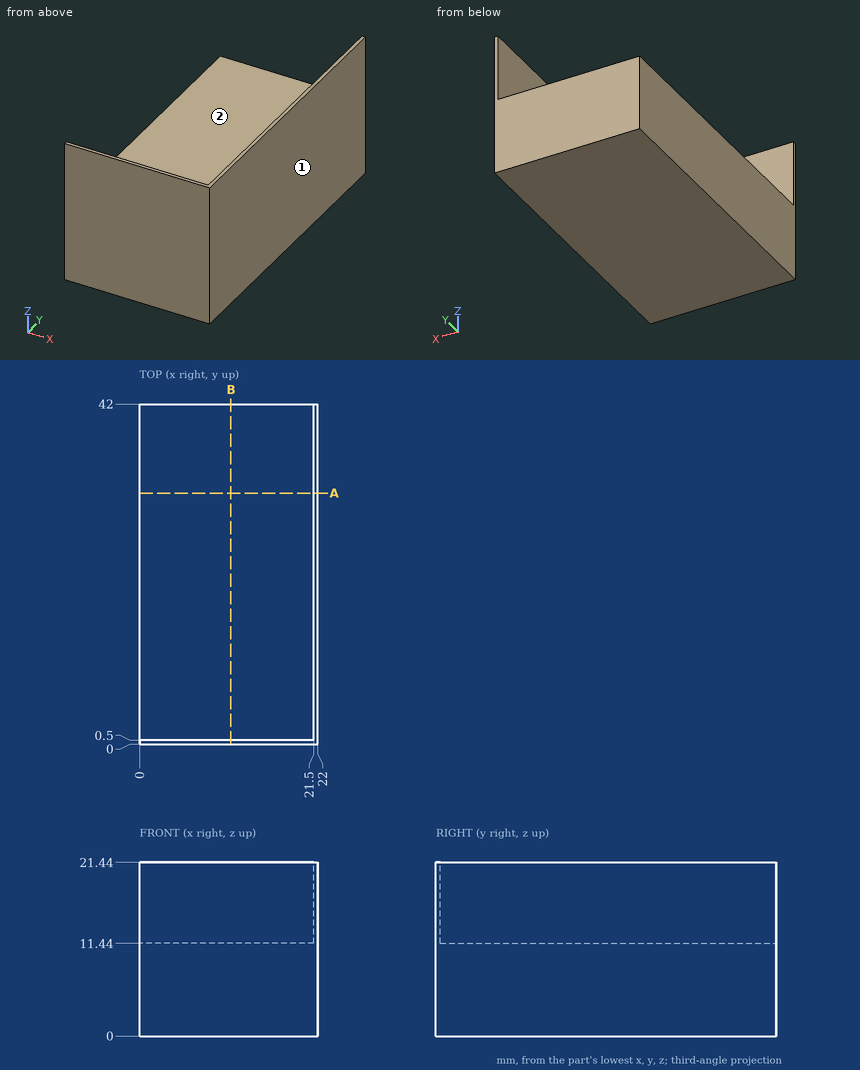
Input: dimensioned drawing with shaded views. Units: mm. Origin: part minimum x, y, z. A direction names the side the tool comes from. Coordinates: 2 decimals unless noted, no trailing zeros. Order: outer loops, then holes, each group sorted by start corner. A loop starts at its lowest first (then second) coordinate and runs counter-clockwise, first axis right, second up. Notation, with made-up numbers: (6.5, 86.5) - (18.5, 86.5) arc R18 cw to (18.5, 93.5) - close; hole circle Ø10 at (67, -11.75). An arc over 180 degrees is marked (long way). One line per item, written item: value.
1) Reachability of the marked faces 1 and 2 from +Z, -Z, +X, -X, +Y, -Y: full face, straight path, thin tool, end or side. Return the list, or none.
Computed values:
face 1: +Z, -Z, +X, +Y, -Y
face 2: +Z, -X, +Y
2) Cut plane B-B on x = 11.25. Output: boundary loops of the cut face in (y, z).
Computed values:
outline: (0, 0) - (42, 0) - (42, 11.44) - (0.5, 11.44) - (0.5, 21.44) - (0, 21.44) - close
3) Contact query for flat-ended pins moving along their axis: pin 1 (4 mm diameter, centred on y = 28, z = 16.5, fed in from -X); pin 2 (8 mm diameter, centred on x = 7, y = 23.5, fed in from +Z); pin 3 (3 mm diameter, centred on x = 15.5, z = 16.5, fed in from +Y); pin 4 (8 mm diameter, centred on y = 6.5, z = 3, fed in from -X). Output: stop coordinate, or through.
Computed values:
pin 1: stops at x = 21.5
pin 2: stops at z = 11.44
pin 3: stops at y = 0.5
pin 4: stops at x = 0
4) Cut plane A-A on y = 31. Output: boundary loops of the cut face in (x, z), plus the area to 3 significant figures.
Computed values:
outline: (0, 0) - (22, 0) - (22, 21.44) - (21.5, 21.44) - (21.5, 11.44) - (0, 11.44) - close
area: 257 mm^2
5) Ray query, line 1 (Z direction, x = 1.75, y = 5.5); line 2 (Y direction, x = 10.5, z = 18.5); line 3 (X direction, y = 34, z = 16.75). Return the intervals inside material, ascending. Write a range as [from, to].
Computed values:
line 1: z = [0, 11.44]
line 2: y = [0, 0.5]
line 3: x = [21.5, 22]
